Here's how the part is built. I have some questions about the finished solid (model axes, mm). Face numbers are marked on the shaded views. A direction names the side the tool comes from. Give positions to 0.01 mm unless a question says otherwise; leave off trailing zeros. Write each loop counter-clockwise with the first axis right and the second up, starting at its lowest first coordinate (ties: lowest second). Pieces come first, ordered by that corner, then holes. Notation, with made-up numbers: (19, 53) -> (43, 53) arc R28 cw to (43, 78) -> close; hole circle Ø6 at (29.25, 6.5). An arc over 180 degrees is marked (long way). Put each result on its own line as item: value. Start each with the question number.
from build123d import *

# Parameters (mm, degrees)
SKETCH1_W               = 44
SKETCH1_H               = 29
SKETCH1_R               = 2.5
BOSS_EXTRUDE1_DEPTH     = 30
CUT_EXTRUDE1_DEPTH      = 25
CUT_EXTRUDE2_DEPTH      = 1
CUT_EXTRUDE2_DEPTH_BACK = 30
SKETCH3_W               = 20
SKETCH3_H               = 7
SKETCH4_R               = 5
CUT_EXTRUDE3_DEPTH      = 3
THICKEN1_T1             = 2
CHAMFER1_SIZE           = 3
CHAMFER2_SIZE           = 4
CUT_EXTRUDE4_DEPTH      = 0.3


with BuildPart() as part:
    # Sketch1 → Boss-Extrude1 (new body)
    with BuildSketch(Plane.XY.offset(794.620141885)):
        with Locations((45.789156386, -208.298939869)):
            Rectangle(SKETCH1_W, SKETCH1_H)
        with Locations((38.789156386, -208.298939869)):
            Circle(SKETCH1_R, mode=Mode.SUBTRACT)
        with Locations((51.789156386, -208.298939869)):
            Circle(SKETCH1_R, mode=Mode.SUBTRACT)
    extrude(amount=BOSS_EXTRUDE1_DEPTH)

    # Sketch2 → Cut-Extrude1 (cut)
    with BuildSketch(Plane.XZ.offset(222.798939869)):
        Polygon((28.289156386, 816.620141885), (48.789156386, 816.620141885), (48.789156386, 806.620141885), (63.289156386, 806.620141885), (63.289156386, 796.620141885), (42.189156386, 796.620141885), (42.189156386, 806.620141885), (28.289156386, 806.620141885), align=None)
    extrude(amount=-CUT_EXTRUDE1_DEPTH, mode=Mode.SUBTRACT)

    # Sketch3 → Cut-Extrude2 (cut, two sides: drawn at the far end of the back side and taken through both)
    with BuildSketch(Plane(origin=(42.189156386, 0, 0), x_dir=(0, 0, -1), z_dir=(1, 0, 0)).offset(-CUT_EXTRUDE2_DEPTH_BACK)):
        with Locations((-806.620141885, -201.298939869)):
            Rectangle(SKETCH3_W, SKETCH3_H)
    extrude(amount=CUT_EXTRUDE2_DEPTH + CUT_EXTRUDE2_DEPTH_BACK, mode=Mode.SUBTRACT)

    # Sketch4 → Cut-Extrude3 (cut)
    with BuildSketch(Plane.XY.offset(824.620141885)):
        with Locations((38.789156386, -208.298939869)):
            Circle(SKETCH4_R)
        with Locations((51.789156386, -208.298939869)):
            Circle(SKETCH4_R)
    extrude(amount=-CUT_EXTRUDE3_DEPTH, mode=Mode.SUBTRACT)

    # Surface-Offset1: a surface, a copy of 1 face of the part
    surface_offset1_1 = part.part.faces().sort_by_distance((45.859348885, -208.298939869, 824.620141885))[0]
    add(Solid.thicken(surface_offset1_1, THICKEN1_T1))

    # Chamfer1
    chamfer1_edges = [part.edges().sort_by_distance(p)[0] for p in [
        (67.789156386, -222.798939869, 810.620141885),
        (23.789156386, -222.798939869, 810.620141885),
        (23.789156386, -193.798939869, 810.620141885),
        (67.789156386, -193.798939869, 810.620141885),
        (67.789156386, -208.298939869, 826.620141885),
        (45.789156386, -193.798939869, 826.620141885),
        (23.789156386, -208.298939869, 826.620141885),
        (45.789156386, -222.798939869, 826.620141885),
    ]]
    chamfer(chamfer1_edges, length=CHAMFER1_SIZE)

    # Chamfer2
    chamfer2_edges = [part.edges().sort_by_distance(p)[0] for p in [
        (42.189156386, -222.798939869, 801.620141885),
        (48.789156386, -222.798939869, 811.620141885),
    ]]
    chamfer(chamfer2_edges, length=CHAMFER2_SIZE)

    # Sketch5 → Cut-Extrude4 (cut)
    with BuildSketch(Plane(origin=(67.789156386, 0, 0), x_dir=(0, 0, -1), z_dir=(1, 0, 0))):
        Polygon((-818.620141885, -210.973121437), (-818.620141885, -209.178249642), (-800.671423936, -209.178249642), (-800.671423936, -201.48594195), (-798.620141885, -201.48594195), (-798.620141885, -210.973121437), align=None)
    extrude(amount=-CUT_EXTRUDE4_DEPTH, mode=Mode.SUBTRACT)


solid = part.part
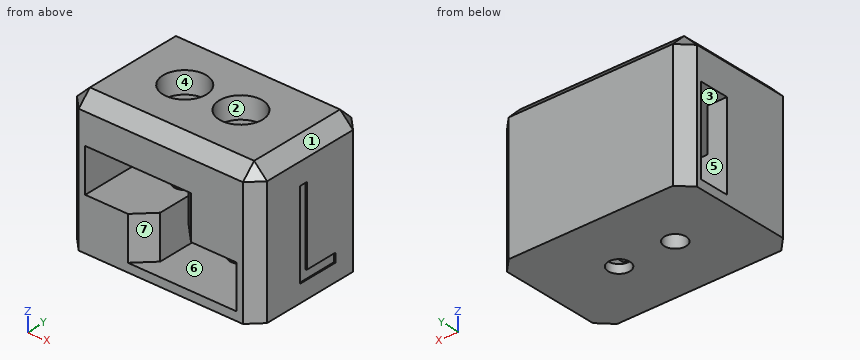
1) Which directions (+Z, -Z, +X, -X, +Y, -Y) give clear straight access to the entire face, cutting with the end or side of a thin tool? Please do the marked faces 4, 5, 6 and 7.
2) I want a section at D-D, the plane z = 815.5. Write out the boundary of the cut face in (x, y), and give its area (3 significant figures).
3) I need wall thicknesses on probe 1 along Y at (x, z) = (52, 822.5); probe 2 along Z at (x, y) = (29, -201.5); probe 3 along Z at (x, y) = (52, -202.5). Which ranges of each line are inside material? Lowest first, please.
4) I want a section at B-B, the plane y = -214.25. Write out the boundary of the cut face in (x, z), and give its area (3 significant figures).
5) Thinking about a two-plate mould opening in Z: for the marked faces 1, 2 and 3, which applies, released by +Z, released by -Z, zero draft, split by the parting line, or undercut?
6) I'm going to push flat-ended pins straight in: pin 1 Ø1.5 at (x, z) = (60, 800) entering from -Y; pin 2 Ø4.5 at (x, y) = (38.79, -208.3) entering from -Z; pin 3 Ø1.5 at (y, z) = (-203, 802.5) entering from -X; pin 4 Ø9 at (x, y) = (51.79, -208.3) entering from +Z. Where does each tip first touch, or does it pass through?
7) I want a section at A-A, the plane z = 804. Write out the boundary of the cut face in (x, y).
8) I want a section at C-C, the plane x = 40.5. Write out the boundary of the cut face in (y, z).
Established:
1. face 4: +Z
1. face 5: -X
1. face 6: none
1. face 7: -Y
2. outline: (23.79, -219.8) -> (26.79, -222.8) -> (28.29, -222.8) -> (28.29, -204.8) -> (23.79, -204.8) -> close; (23.79, -197.8) -> (48.79, -197.8) -> (48.79, -218.8) -> (52.79, -222.8) -> (64.79, -222.8) -> (67.79, -219.8) -> (67.79, -210.97) -> (67.49, -210.97) -> (67.49, -209.18) -> (67.79, -209.18) -> (67.79, -196.8) -> (64.79, -193.8) -> (26.79, -193.8) -> (23.79, -196.8) -> close; hole circle Ø5 at (51.79, -208.3)
2. area: 686 mm2
3. probe 1: y = -222.8 to -213.29, -203.3 to -193.8
3. probe 2: z = 794.62 to 796.62, 816.62 to 826.62
3. probe 3: z = 794.62 to 796.62, 806.62 to 826.62
4. outline: (23.79, 794.62) -> (67.79, 794.62) -> (67.79, 823.62) -> (64.79, 826.62) -> (26.79, 826.62) -> (23.79, 823.62) -> close; hole (28.29, 806.62) -> (42.19, 806.62) -> (42.19, 796.62) -> (63.29, 796.62) -> (63.29, 806.62) -> (48.79, 806.62) -> (48.79, 816.62) -> (28.29, 816.62) -> close
4. area: 983 mm2
5. face 1: released by +Z
5. face 2: zero draft
5. face 3: undercut
6. pin 1: stops at y = -197.8
6. pin 2: passes through
6. pin 3: stops at x = 63.29
6. pin 4: stops at z = 821.62
7. outline: (23.79, -219.8) -> (26.79, -222.8) -> (38.19, -222.8) -> (42.19, -218.8) -> (42.19, -204.8) -> (23.79, -204.8) -> close; (23.79, -197.8) -> (63.29, -197.8) -> (63.29, -222.8) -> (64.79, -222.8) -> (67.79, -219.8) -> (67.79, -210.97) -> (67.49, -210.97) -> (67.49, -209.18) -> (67.79, -209.18) -> (67.79, -196.8) -> (64.79, -193.8) -> (26.79, -193.8) -> (23.79, -196.8) -> close; hole circle Ø5 at (38.79, -208.3)
8. outline: (-222.8, 794.62) -> (-210.12, 794.62) -> (-210.12, 806.62) -> (-220.49, 806.62) -> (-220.49, 796.62) -> (-222.8, 796.62) -> close; (-222.8, 816.62) -> (-210.12, 816.62) -> (-210.12, 821.62) -> (-213, 821.62) -> (-213, 826.62) -> (-219.8, 826.62) -> (-222.8, 823.62) -> close; (-206.48, 794.62) -> (-193.8, 794.62) -> (-193.8, 823.62) -> (-196.8, 826.62) -> (-203.6, 826.62) -> (-203.6, 821.62) -> (-206.48, 821.62) -> (-206.48, 816.62) -> (-197.8, 816.62) -> (-197.8, 796.62) -> (-204.8, 796.62) -> (-204.8, 806.62) -> (-206.48, 806.62) -> close
